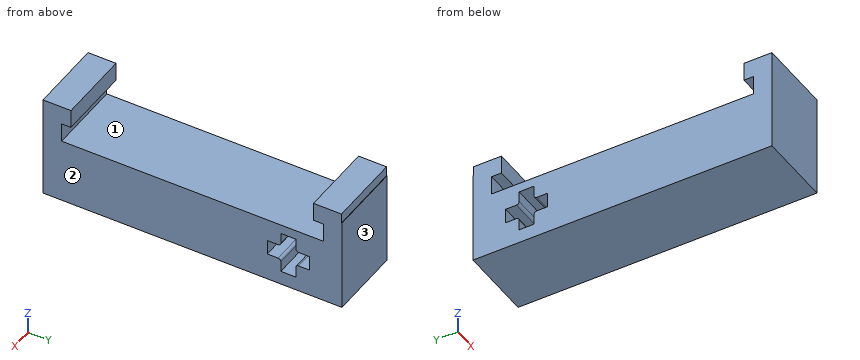
from build123d import *

# Parameters (mm, degrees)
BOX005_W     = 8
BOX005_H     = 3
BOX005_DEPTH = 2
BOX001_W     = 80
BOX001_H     = 4.5
BOX001_DEPTH = 1.6
BOX_W        = 80
BOX_H        = 4.5
BOX_DEPTH    = 1.6
BOX002_W     = 8
BOX002_H     = 7.5
BOX002_DEPTH = 7
FILLET_R     = 0.3
BOX003_W     = 8
BOX003_H     = 2
BOX003_DEPTH = 10
BOX006_W     = 8
BOX006_H     = 21
BOX006_DEPTH = 7
BOX007_W     = 8
BOX007_H     = 3
BOX007_DEPTH = 2
BOX008_W     = 8
BOX008_H     = 2
BOX008_DEPTH = 10


with BuildPart() as cube005:
    # Box005 → Box005 (new body)
    with BuildSketch(Plane(origin=(0, 2.7, 5.3), x_dir=(1, 0, 0), z_dir=(0, 0, 1))):
        with Locations((4, 1.5)):
            Rectangle(BOX005_W, BOX005_H)
    extrude(amount=BOX005_DEPTH)


with BuildPart() as cube001:
    # Box001 → Box001 (new body)
    with BuildSketch(Plane(origin=(0, 0.8, -2.25), x_dir=(1, 0, 0), z_dir=(0, -1, 0))):
        with Locations((40, 2.25)):
            Rectangle(BOX001_W, BOX001_H)
    extrude(amount=BOX001_DEPTH)


with BuildPart() as fusion:
    # Box → Box (new body)
    with BuildSketch(Plane(origin=(0, -2.25, -0.8), x_dir=(1, 0, 0), z_dir=(0, 0, 1))):
        with Locations((40, 2.25)):
            Rectangle(BOX_W, BOX_H)
    extrude(amount=BOX_DEPTH)

    # Fusion: union Cube001
    add(cube001.part)


with BuildPart() as fusion_1:
    # Fusion placement: moved
    add(fusion.part.moved(Location((-5, 0, 0))))


with BuildPart() as fillet_body:
    # Box002 → Box002 (new body)
    with BuildSketch(Plane(origin=(0, -3.75, -3.75), x_dir=(1, 0, 0), z_dir=(0, 0, 1))):
        with Locations((4, 3.75)):
            Rectangle(BOX002_W, BOX002_H)
    extrude(amount=BOX002_DEPTH)

    # Cut: cut Fusion
    add(fusion_1.part, mode=Mode.SUBTRACT)

    # Fillet
    fillet_edges = [fillet_body.edges().sort_by_distance(p)[0] for p in [
        (4, -0.8, 0.8),
        (4, -0.8, -0.8),
        (4, 0.8, -0.8),
        (4, 0.8, 0.8),
    ]]
    fillet(fillet_edges, radius=FILLET_R)


with BuildPart() as fusion001:
    # Box003 → Box003 (new body)
    with BuildSketch(Plane(origin=(0, 3.75, -3.75), x_dir=(1, 0, 0), z_dir=(0, 0, 1))):
        with Locations((4, 1)):
            Rectangle(BOX003_W, BOX003_H)
    extrude(amount=BOX003_DEPTH)

    # Fusion001: union Cube005, Fillet body
    add(cube005.part)
    add(fillet_body.part)


with BuildPart() as fusion002:
    # Box006 → Box006 (new body)
    with BuildSketch(Plane(origin=(0, -24.3, -3.75), x_dir=(1, 0, 0), z_dir=(0, 0, 1))):
        with Locations((4, 10.5)):
            Rectangle(BOX006_W, BOX006_H)
    extrude(amount=BOX006_DEPTH)

    # Fusion002: union Fusion001
    add(fusion001.part)


with BuildPart() as cube007:
    # Box007 → Box007 (new body)
    with BuildSketch(Plane(origin=(0, -26.3, 5.3), x_dir=(1, 0, 0), z_dir=(0, 0, 1))):
        with Locations((4, 1.5)):
            Rectangle(BOX007_W, BOX007_H)
    extrude(amount=BOX007_DEPTH)


with BuildPart() as fusion004:
    # Box008 → Box008 (new body)
    with BuildSketch(Plane(origin=(0, -26.3, -3.75), x_dir=(1, 0, 0), z_dir=(0, 0, 1))):
        with Locations((4, 1)):
            Rectangle(BOX008_W, BOX008_H)
    extrude(amount=BOX008_DEPTH)

    # Fusion003: union Cube007
    add(cube007.part)

    # Fusion004: union Fusion002
    add(fusion002.part)


solid = fusion004.part
Model file for the job. Use its own axes, mm. Face numbers are marked on the shaded views. Coordinates: 2 decimals unless noted, no trailing zeros. Order: outer loops, then holes, each group sorted by start corner. A loop starts at its lowest first (then second) coordinate and runs counter-clockwise, first axis right, second up. Notation, with made-up numbers: (73, 19.5) -> (109, 19.5) arc R16 ccw to (109, 27.5) -> close; hole circle Ø6 at (30.5, -38). An arc over 180 degrees is marked (long way). Return JSON: item names as keys, results as strings. Group by question number.
Item 1: Saw through at A-A on z = 4.75. Write the cut outline in (x, y), then the cut area to 3 significant figures.
Item 2: Saw through at C-C on z = -1.5. Write the cut outline in (x, y).
Item 3: Wall check: line 1 along Z through (x, y) = (3, 2); line 2 along Y through (x, z) = (7, 4); line 3 along Y through (x, z) = (7, 1.5). Give the ranges that are in metal, low to high. Write a range as [from, to].
Item 4: Pull direction Y, two halves, no side cores. Call the marked faces 1, 2 and 3: pulls with the +Y half, pulls with the -Y half, needs draft (parallel to the pull), parting line crosses it, or undercut.
Item 5: Saw through at D-D on y = -22.5. Write the cut outline in (x, z), then the cut area to 3 significant figures.
Item 6: Flat gauge pin, fed straight in: P1, Ø1.3, axis at x = 5, y = 1.5, coming from the +Z side. Where does the tip first touch, or does it go through?
Values found:
{
 "1": {"outline": "(0, -26.3) -> (8, -26.3) -> (8, -24.3) -> (0, -24.3) -> close; (0, 3.75) -> (8, 3.75) -> (8, 5.75) -> (0, 5.75) -> close", "area": "32.0 mm2"},
 "2": {"outline": "(0, -26.3) -> (8, -26.3) -> (8, -0.8) -> (0, -0.8) -> close; (0, 0.8) -> (8, 0.8) -> (8, 5.75) -> (0, 5.75) -> close"},
 "3": {"line 1": "z = [-3.75, -0.8], [0.8, 3.25]", "line 2": "y = [-26.3, -24.3], [3.75, 5.75]", "line 3": "y = [-26.3, -0.8], [0.8, 5.75]"},
 "4": {"face 1": "undercut", "face 2": "needs draft", "face 3": "pulls with the +Y half"},
 "5": {"outline": "(0, -3.75) -> (8, -3.75) -> (8, 3.25) -> (0, 3.25) -> close", "area": "56.0 mm2"},
 "6": {"P1": "stops at z = 3.25"}
}
